from build123d import *

# Parameters (mm, degrees)
SKETCH2_R           = 8
BOSS_EXTRUDE1_DEPTH = 100
SKETCH3_R           = 5.25
CUT_EXTRUDE1_DEPTH  = 21
CUT_EXTRUDE2_START  = -5.5
SKETCH4_R           = 5.25
CUT_EXTRUDE2_DEPTH  = 5.5


with BuildPart() as part:
    # Sketch2 → Boss-Extrude1 (new body)
    with BuildSketch(Plane.XY):
        Circle(SKETCH2_R)
    extrude(amount=BOSS_EXTRUDE1_DEPTH)

    # Sketch3 → Cut-Extrude1 (cut)
    with BuildSketch(Plane(origin=(0, 0, 0), x_dir=(-1, 0, 0), z_dir=(0, 0, -1))):
        Circle(SKETCH3_R)
    extrude(amount=-CUT_EXTRUDE1_DEPTH, mode=Mode.SUBTRACT)

    # Sketch4 → Cut-Extrude2 (cut)
    with BuildSketch(Plane.XY.offset(100).offset(CUT_EXTRUDE2_START)):
        with Locations(Location((0, 0, 0), (0, 0, 180))):
            Circle(SKETCH4_R)
    extrude(amount=CUT_EXTRUDE2_DEPTH, mode=Mode.SUBTRACT)


solid = part.part
The model under review builds one solid part; all positions refer to its coordinate system, in mm. A direction names the side the tool comes from. Coordinates: 2 decimals unless noted, no trailing zeros. Write each loop counter-clockwise with the first axis right and the second up, starting at its lowest first coordinate (ties: lowest second). Pieces come first, ordered by that corner, then holes. Notation, with made-up numbers: (78.5, 40.25) - (97.5, 40.25) arc R30 ccw to (97.5, 75.25) - close; hole circle Ø9 at (5, -17). An arc over 180 degrees is marked (long way). Answer as a JSON object with one key per item and string values. Group by question number.
1. Machinability: for faces 1 (the face through (-5, 1.6, 10.4)), 2 (the face through (-5, -1.6, 97.2)), 3 (the face through (5.2, -1.7, 100)), which of the approach directions +Z, -Z, +X, -X, +Y, -Y give a long, thin tool a straight path to every point of the face, cutting with its end or side? Answer none if there is none.
2. Add section C-C (z = 11). Give the boundary of the cut face in (x, y).
3. To check wall thickness, follow probe 1 along Y at (x, z) = (0, 4.5); probe 2 along Z at (x, y) = (4.5, 2.25); probe 3 along Y at (x, z) = (-1.25, 62.5). State the ranges of each line that lie inside material, in increasing order.
4. Clearance check with flat-ended pins moving along their axes: pin 1 Ø3 at (x, y) = (-2.5, 0.5) entering from +Z; pin 2 Ø1.5 at (y, z) = (5, 59.5) entering from -X; pin 3 Ø2 at (y, z) = (2.5, 78.5) entering from +X. State where each tip first meets the part, or that it passes through.
5. Add section D-D (z = 91.5). Give the boundary of the cut face in (x, y), plus the area to 3 significant figures.
6. Add section A-A (y = 0). Give the boundary of the cut face in (x, z).
Findings:
{
 "1": {"face 1": "-Z", "face 2": "+Z", "face 3": "+Z, +X, -X, +Y, -Y"},
 "2": {"outline": "circle Ø16 at (0, 0); hole circle Ø10.5 at (0, 0)"},
 "3": {"probe 1": "-8 to -5.25, 5.25 to 8", "probe 2": "21 to 94.5", "probe 3": "-7.9 to 7.9"},
 "4": {"pin 1": "z = 94.5", "pin 2": "x = -6.78", "pin 3": "x = 7.86"},
 "5": {"outline": "circle Ø16 at (0, 0)", "area": "201 mm²"},
 "6": {"outline": "(-8, 0) - (-5.25, 0) - (-5.25, 21) - (5.25, 21) - (5.25, 0) - (8, 0) - (8, 100) - (5.25, 100) - (5.25, 94.5) - (-5.25, 94.5) - (-5.25, 100) - (-8, 100) - close"}
}
